Read the model definition and answer for the solid it produces. Units are mm, in the model's axes. A direction names the side the tool comes from. Round coordinates to 2 decimals unless told otherwise and drop trailing zeros. Write each loop counter-clockwise with the first axis right and the second up, starting at its lowest first coordinate (ties: lowest second). Pieces come first, ordered by that corner, then holes. Notation, with made-up numbers: (80.25, 24) -> (132.25, 24) arc R14 ccw to (132.25, 29) -> close; hole circle Ø5 at (40.5, -18). An arc over 180 degrees is marked (long way). Return JSON: item names as keys, results as strings.
from build123d import *

# Parameters (mm, degrees)
SKETCH1_W           = 65
SKETCH1_H           = 95
PUMP_HEAD_DEPTH     = 100
MOTOR_START         = 65
SKETCH2_R           = 40
MOTOR_DEPTH         = 85
INLET_PORT_START    = -12
SKETCH3_R           = 6
INLET_PORT_DEPTH    = 12
INLET_SOCKET_START  = -12
SKETCH4_R           = 3.2
INLET_SOCKET_DEPTH  = 10
OUTLET_PORT_START   = -12
SKETCH5_R           = 6
OUTLET_PORT_DEPTH   = 12
OUTLET_SOCKET_START = -12
SKETCH6_R           = 3.2
OUTLET_SOCKET_DEPTH = 10
CABLE_STUB_START    = 150
SKETCH7_R           = 3
CABLE_STUB_DEPTH    = 10


with BuildPart() as part:
    # Sketch1 → Pump_Head (new body)
    with BuildSketch(Plane(origin=(0, 0, 0), x_dir=(1, 0, 0), z_dir=(0, 1, 0))):
        with Locations((32.5, 0)):
            Rectangle(SKETCH1_W, SKETCH1_H)
    extrude(amount=PUMP_HEAD_DEPTH)

    # Sketch2 → Motor (add)
    with BuildSketch(Plane(origin=(0, 0, 0), x_dir=(0, 0, -1), z_dir=(1, 0, 0)).offset(MOTOR_START)):
        with Locations((0, 50)):
            Circle(SKETCH2_R)
    extrude(amount=MOTOR_DEPTH)

    # Sketch3 → Inlet_Port (add)
    with BuildSketch(Plane(origin=(0, 0, 0), x_dir=(0, 0, -1), z_dir=(1, 0, 0)).offset(INLET_PORT_START)):
        with Locations((0, 30)):
            Circle(SKETCH3_R)
    extrude(amount=INLET_PORT_DEPTH)

    # Sketch4 → Inlet_Socket (cut)
    with BuildSketch(Plane(origin=(0, 0, 0), x_dir=(0, 0, -1), z_dir=(1, 0, 0)).offset(INLET_SOCKET_START)):
        with Locations((0, 30)):
            Circle(SKETCH4_R)
    extrude(amount=INLET_SOCKET_DEPTH, mode=Mode.SUBTRACT)

    # Sketch5 → Outlet_Port (add)
    with BuildSketch(Plane(origin=(0, 0, 0), x_dir=(0, 0, -1), z_dir=(1, 0, 0)).offset(OUTLET_PORT_START)):
        with Locations((0, 70)):
            Circle(SKETCH5_R)
    extrude(amount=OUTLET_PORT_DEPTH)

    # Sketch6 → Outlet_Socket (cut)
    with BuildSketch(Plane(origin=(0, 0, 0), x_dir=(0, 0, -1), z_dir=(1, 0, 0)).offset(OUTLET_SOCKET_START)):
        with Locations((0, 70)):
            Circle(SKETCH6_R)
    extrude(amount=OUTLET_SOCKET_DEPTH, mode=Mode.SUBTRACT)

    # Sketch7 → Cable_Stub (add)
    with BuildSketch(Plane(origin=(0, 0, 0), x_dir=(0, 0, -1), z_dir=(1, 0, 0)).offset(CABLE_STUB_START)):
        with Locations((0, 50)):
            Circle(SKETCH7_R)
    extrude(amount=CABLE_STUB_DEPTH)


solid = part.part
Item 1: Flat-ended cylindrical pins translate along their axes: pin 1 (6 mm diameter, centred on y = 30, z = 0, fed in from +X); pin 2 (1 mm diameter, centred on x = 123, z = -12.5, fed in from -Y); pin 3 (1 mm diameter, centred on y = 39.5, z = -11, fed in from -X). Find the tip coordinate at first contact, or state that the pin passes through.
Worked answers:
{"pin 1": "stops at x = 150", "pin 2": "stops at y = 11.84", "pin 3": "stops at x = 0"}
Item 2: Section C-C (x = 125) is taken. Give the vertices of the cut face in (y, z), then the cut area to 3 significant figures.
Worked answers:
{"outline": "circle Ø80 at (50, 0)", "area": "5,030 mm2"}
Item 3: Section A-A (y = 50) is taken. Give the vertices of the cut face in (x, z), then the cut area to 3 significant figures.
Worked answers:
{"outline": "(0, -47.5) -> (65, -47.5) -> (65, -40) -> (150, -40) -> (150, -3) -> (160, -3) -> (160, 3) -> (150, 3) -> (150, 40) -> (65, 40) -> (65, 47.5) -> (0, 47.5) -> close", "area": "13,000 mm2"}
Item 4: Straight lines are drawn through the part: L1, parallel to Y at x = -9, z = 0; L2, parallel to X at y = 64, z = 18; L3, parallel to X at y = 23, z = 44. For each, find the intervals that lie inside material, in ascending order. Write a range as [from, to].
Worked answers:
{"L1": "y = [24, 26.8], [33.2, 36], [64, 66.8], [73.2, 76]", "L2": "x = [0, 150]", "L3": "x = [0, 65]"}
Item 5: Section D-D (z = -24) is taken. Give the vertices of the cut face in (x, y).
Worked answers:
{"outline": "(0, 0) -> (65, 0) -> (65, 18) -> (150, 18) -> (150, 82) -> (65, 82) -> (65, 100) -> (0, 100) -> close"}
Item 6: A tool of negligible diameter and unlimited length cuts with its end or side. For faces 1 (the cylindrical face through (106.9, 10.95, 8.67)), 2 (the flat face through (-12, 67, -3)), 3 (the cylindrical face through (-6.084, 24.143, 1.301)), from which of +Z, -Z, +X, -X, +Y, -Y can it reach the whole face along a straight path? Write none if from no direction.
Worked answers:
{"face 1": "+X", "face 2": "+Z, -Z, -X, +Y, -Y", "face 3": "-X"}
Item 7: Section B-B (z = 0) is taken. Give the vertices of the cut face in (x, y), then the cut area to 3 significant figures.
Worked answers:
{"outline": "(-12, 24) -> (0, 24) -> (0, 0) -> (65, 0) -> (65, 10) -> (150, 10) -> (150, 47) -> (160, 47) -> (160, 53) -> (150, 53) -> (150, 90) -> (65, 90) -> (65, 100) -> (0, 100) -> (0, 76) -> (-12, 76) -> (-12, 73.2) -> (-2, 73.2) -> (-2, 66.8) -> (-12, 66.8) -> (-12, 64) -> (0, 64) -> (0, 36) -> (-12, 36) -> (-12, 33.2) -> (-2, 33.2) -> (-2, 26.8) -> (-12, 26.8) -> close", "area": "13,500 mm2"}
Item 8: For a pull along Z with two mould halves and no side action, classify faces 4 (the cylindrical face through (155, 53, 0)), 5 (the cylindrical face through (-7.07, 67.161, -1.477)), 6 (the flat face through (-2, 30, 0)), 7 (the flat face through (32, 0, -1)) as released by +Z, released by -Z, zero draft, split by the parting line, or undercut.
Worked answers:
{"face 4": "split by the parting line", "face 5": "undercut", "face 6": "undercut", "face 7": "zero draft"}
